Work out the finished part from the listing and answer in its coordinate system (mm). A direction names the side the tool comes from. Coordinates: 2 decimals unless noted, no trailing zeros. Write each loop counter-clockwise with the first axis right and the second up, starting at its lowest first coordinate (ties: lowest second). Pieces come first, ordered by that corner, then holes. Notation, with made-up numbers: M 72,-34.5 L 105,-34.5 A14 cw 105,-28.5 Z; hole C 65.5,-12 d10. An arc over 180 degrees is marked long. Use CSV: the item, a comma, the result in double quotes.
from build123d import *

# Parameters (mm, degrees)
F0_W     = 101.6
F0_H     = 76.2
F1_DEPTH = 152.4
F2_W     = 76.2
F2_H     = 25.4
F3_DEPTH = 50.8
F4_R     = 5.08


with BuildPart() as f1:
    # F0 (on Front) → F1 (new body)
    with BuildSketch(Plane.XZ):
        with Locations((10.387156, -20.946899)):
            Rectangle(F0_W, F0_H)
    extrude(amount=F1_DEPTH)

    # F2 (on face) → F3 (cut)
    with BuildSketch(Plane.XY.offset(17.153101)):
        with Locations((10.387156, -22.86)):
            Rectangle(F2_W, F2_H)
        with Locations((10.387156, -58.42)):
            Rectangle(F2_W, F2_H)
        with Locations((10.387156, -93.98)):
            Rectangle(F2_W, F2_H)
        with Locations((10.387156, -129.54)):
            Rectangle(F2_W, F2_H)
    extrude(amount=-F3_DEPTH, mode=Mode.SUBTRACT)

    # F4
    f4_edges = [f1.edges().sort_by_distance(p)[0] for p in [
        (61.187156, 0, -20.946899),
        (10.387156, 0, -59.046899),
        (10.387156, 0, 17.153101),
        (-40.412844, 0, -20.946899),
    ]]
    fillet(f4_edges, radius=F4_R)


solid = f1.part
Item 1: Given pin 1 (7.5 mm diameter, centred on x = -1.5, y = -128.5, fed in from +Z), flat-ended and moving along its own axis, determine where the tip first touches the part or whether it passes through.
Answer:
pin 1,"stops at z = -33.65"
Item 2: For a pull along X with two mould halves and no side action, classify faces 1 (the face through (59.66, -1.45, -20.41)), 2 (the face through (10, -35.56, -8)), 3 (the face through (10, -45.72, -8)), 4 (the face through (10, -78, -59.047)) as released by +X, released by -X, zero draft, split by the parting line, or undercut.
Answer:
face 1,"released by +X"
face 2,"undercut"
face 3,"undercut"
face 4,"zero draft"
Item 3: The part is cut by section B-B (y = -88.5). Write down the section's boundary in (x, z), then the cut area to 3 significant figures.
Answer:
outline,"M -40.41,-59.05 L 61.19,-59.05 L 61.19,17.15 L 48.49,17.15 L 48.49,-33.65 L -27.71,-33.65 L -27.71,17.15 L -40.41,17.15 Z"
area,"3,870 mm2"
Item 4: The part is cut by section A-A (z = 3.5). Write down the section's boundary in (x, y), then the cut area to 3 significant figures.
Answer:
outline,"M -40.41,-152.4 L 61.19,-152.4 L 61.19,-5.08 A5.08 ccw 56.11,0 L -35.33,0 A5.08 ccw -40.41,-5.08 Z; hole M -27.71,-142.24 L 48.49,-142.24 L 48.49,-116.84 L -27.71,-116.84 Z; hole M -27.71,-106.68 L 48.49,-106.68 L 48.49,-81.28 L -27.71,-81.28 Z; hole M -27.71,-71.12 L 48.49,-71.12 L 48.49,-45.72 L -27.71,-45.72 Z; hole M -27.71,-35.56 L 48.49,-35.56 L 48.49,-10.16 L -27.71,-10.16 Z"
area,"7,730 mm2"
Item 5: The part is cut by section C-C (x = -14). Write down the section's boundary in (y, z).
Answer:
outline,"M -152.4,-59.05 L -5.08,-59.05 A5.08 ccw 0,-53.97 L 0,12.07 A5.08 ccw -5.08,17.15 L -10.16,17.15 L -10.16,-33.65 L -35.56,-33.65 L -35.56,17.15 L -45.72,17.15 L -45.72,-33.65 L -71.12,-33.65 L -71.12,17.15 L -81.28,17.15 L -81.28,-33.65 L -106.68,-33.65 L -106.68,17.15 L -116.84,17.15 L -116.84,-33.65 L -142.24,-33.65 L -142.24,17.15 L -152.4,17.15 Z"
Item 6: Consider probe 1 along Y at (x, z) = (34, 0.5); probe 2 along X at (y, z) = (-67, 9); probe 3 along Z at (x, y) = (-25.5, -125.5). Determine where each line is inside the solid, lowest interval first.
Answer:
probe 1,"y = -152.4 to -142.24, -116.84 to -106.68, -81.28 to -71.12, -45.72 to -35.56, -10.16 to 0"
probe 2,"x = -40.41 to -27.71, 48.49 to 61.19"
probe 3,"z = -59.05 to -33.65"
Item 7: A tool of negligible diameter and unlimited length cuts with its end or side. For faces 5 (the face through (-40.413, -78, -21)), 6 (the face through (10, -23, -33.647)), from which of +Z, -Z, +X, -X, +Y, -Y can it reach the whole face along a straight path? Write none if from no direction.
Answer:
face 5,"+Z, -Z, -X, +Y, -Y"
face 6,"+Z"
